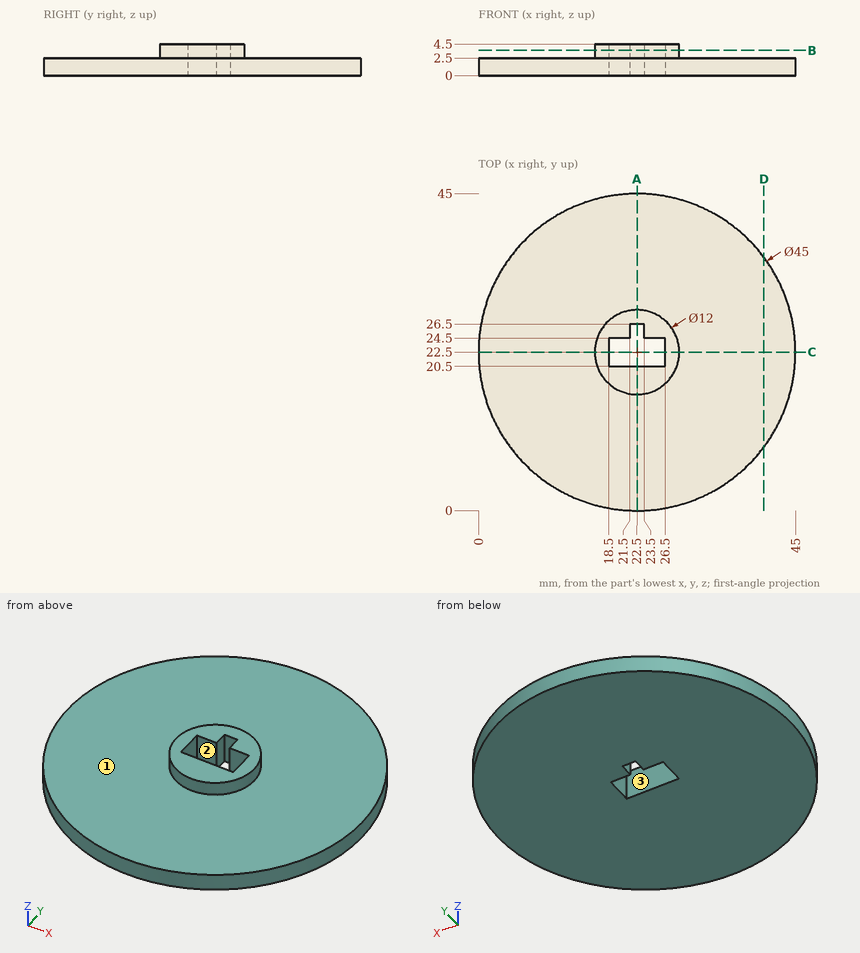
Geometry: see drawing. Coordinates: mm, zero at the bounding-box minimum. Give positions to 0.01 mm unless a question says otherwise; leave off trailing zeros. Write each loop counter-clockwise with the first axis right and the second up, starting at its lowest first coordinate (ties: lowest second). Pieces come first, ordered by that corner, then holes. Notation, with made-up numbers: (9, 1.5) -> (28, 1.5) arc R33 ccw to (28, 29.5) -> close; hole circle Ø7 at (62.25, 18.25). An arc over 180 degrees is marked (long way). Use one line per item in the form item = value. Start each with the question number.
1) Pin query (flat end, axial travel): pin 1 (1.5 mm diameter, centred on x = 24.5, z = 1.5, fed in from -Y); pin 2 (1.5 mm diameter, centred on x = 6, y = 29, fed in from +Z); pin 3 (1 mm diameter, centred on x = 13.5, z = 2, fed in from +Y). Return the tip coordinate at first contact, or that it passes through.
2) Section query D-D on x = 40.5. Return the cut outline in (y, z), then the cut area to 3 significant figures.
3) Section query C-C on y = 22.5. Return the cut outline in (x, z).
4) Ray query, probe 1 along Z at (x, y) = (16, 35.5); probe 2 along Y at (x, z) = (20.5, 2.6); probe 3 along X at (y, z) = (25, 3.25). Return the intervals inside material, ascending. Write a range as from..to.
5) Section query A-A on x = 22.5. Return the cut outline in (y, z), then the cut area to 4 significant figures.
6) Draft query along Y for the marked faces 1, 2 and 3. Return one class per face: pulls with the +Y half, pulls with the -Y half, needs draft (parallel to the pull), parting line crosses it, or undercut.
7) Section query B-B on z = 3.6. Return the cut outline in (x, y), then the cut area to 3 significant figures.
Outcome:
q1.pin_1 = 0.03
q1.pin_2 = 2.5
q1.pin_3 = 43.33
q2.outline = (9, 0) -> (36, 0) -> (36, 2.5) -> (9, 2.5) -> close
q2.area = 67.5 mm^2
q3.outline = (0, 0) -> (18.5, 0) -> (18.5, 4.5) -> (16.5, 4.5) -> (16.5, 2.5) -> (0, 2.5) -> close; (26.5, 0) -> (45, 0) -> (45, 2.5) -> (28.5, 2.5) -> (28.5, 4.5) -> (26.5, 4.5) -> close
q4.probe_1 = 0..2.5
q4.probe_2 = 16.84..20.5, 24.5..28.16
q4.probe_3 = 17.05..21.5, 23.5..27.95
q5.outline = (0, 0) -> (20.5, 0) -> (20.5, 4.5) -> (16.5, 4.5) -> (16.5, 2.5) -> (0, 2.5) -> close; (26.5, 0) -> (45, 0) -> (45, 2.5) -> (28.5, 2.5) -> (28.5, 4.5) -> (26.5, 4.5) -> close
q5.area = 109.5 mm^2
q6.face_1 = needs draft
q6.face_2 = undercut
q6.face_3 = undercut
q7.outline = circle Ø12 at (22.5, 22.5); hole (18.5, 20.5) -> (26.5, 20.5) -> (26.5, 24.5) -> (23.5, 24.5) -> (23.5, 26.5) -> (21.5, 26.5) -> (21.5, 24.5) -> (18.5, 24.5) -> close
q7.area = 77.1 mm^2
